from build123d import *

# Parameters (mm, degrees)
SKETCH_1_R          = 7.5
EXTRUDE_1_DEPTH     = 20
SKETCH_2_R          = 3.5
CUT_EXTRUDE_1_DEPTH = 4
SKETCH_3_R          = 1.75
CUT_EXTRUDE_2_DEPTH = 14
SKETCH_4_R          = 1.4
CUT_EXTRUDE_3_DEPTH = 14
SKETCH_5_W          = 18
SKETCH_5_H          = 5
CUT_EXTRUDE_4_DEPTH = 4


with BuildPart() as part:
    # Эскиз1 → Бобышка-Вытянуть1 (new body)
    with BuildSketch(Plane.XY):
        Circle(SKETCH_1_R)
    extrude(amount=EXTRUDE_1_DEPTH)

    # Эскиз2 → Вырез-Вытянуть1 (cut)
    with BuildSketch(Plane.XY.offset(20)):
        Circle(SKETCH_2_R)
    extrude(amount=-CUT_EXTRUDE_1_DEPTH, mode=Mode.SUBTRACT)

    # Эскиз3 → Вырез-Вытянуть2 (cut)
    with BuildSketch(Plane(origin=(0, 0, 0), x_dir=(-1, 0, 0), z_dir=(0, 0, -1))):
        Circle(SKETCH_3_R)
    extrude(amount=-CUT_EXTRUDE_2_DEPTH, mode=Mode.SUBTRACT)

    # Эскиз4 → Вырез-Вытянуть3 (cut)
    with BuildSketch(Plane(origin=(0, 0, 0), x_dir=(1, 0, 0), z_dir=(0, 1, 0))):
        with Locations(Location((0, -7, 0), (0, 0, 270))):
            Circle(SKETCH_4_R)
    extrude(amount=-CUT_EXTRUDE_3_DEPTH, mode=Mode.SUBTRACT)

    # Эскиз5 → Вырез-Вытянуть4 (cut)
    with BuildSketch(Plane.XY.offset(20)):
        Rectangle(SKETCH_5_W, SKETCH_5_H)
    extrude(amount=-CUT_EXTRUDE_4_DEPTH, mode=Mode.SUBTRACT)


solid = part.part
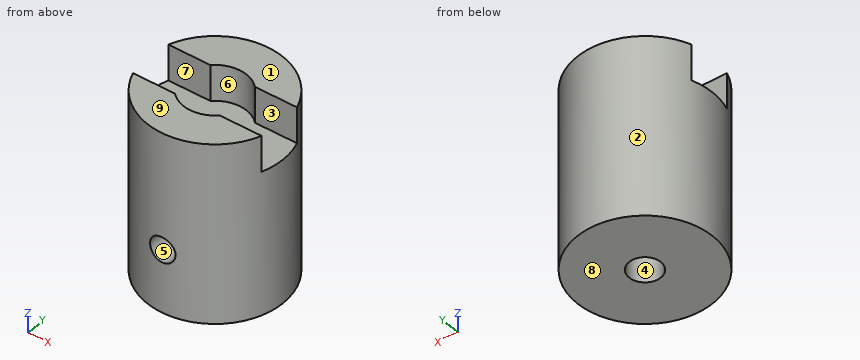
Can you work these out from the model? Positions are in its coordinate system, mm. Face numbers are marked on the shaded views. A direction names the side the tool comes from. Give positions to 0.01 mm unless a question says otherwise; leave off trailing zeros. Write each loop counter-clockwise with the first axis right and the second up, starting at its lowest first coordinate (ties: lowest second). Pieces come first, ordered by that corner, then holes. Notation, with made-up numbers: (53.25, 22) -> (109.25, 22) arc R22 cw to (109.25, 46) -> close; hole circle Ø9 at (55, -6.75). An arc over 180 degrees is marked (long way). Answer as a JSON object with one key per item and string values. Group by question number.
Item 1: For the marked faces 5, 6, 7, 8 and 9, which set-ups out of +Z, -Z, +X, -X, +Y, -Y let a thin tool reach every point of the face, with its end or its side?
Item 2: Suppose I cut it at D-D (x = 6.25). Please give me the cut outline in (y, z), plus the area to 3 significant figures.
Item 3: I'm going to push flat-ended pins straight in: P1, Ø4, axis at x = -2.5, y = 3.5, coming from the -Z side; P2, Ø1, axis at x = 2.5, z = 9.5, coming from the +Y side; P3, Ø2, axis at x = -5, z = 17.5, coming from the -Y side; P4, Ø3, axis at x = -5, z = 17, coming from the +Y side. Where does each tip first touch, or does it pass through?
Item 4: Suppose I cut it at B-B (y = -6). Please give me the cut outline in (x, z).
Item 5: Suppose I cut it at C-C (y = 0). Please give me the cut outline in (x, z), plus the area to 3 significant figures.
Item 6: Please list where these lines run through material, in increasing order: line 1 (Y direction, x = 2.5, z = 18.25); line 2 (Z direction, x = -5, y = -2); line 3 (Z direction, x = 1, y = -4.5). Write a range as [from, to].
Item 7: Suppose I cut it at A-A (x = 0). Please give me the cut outline in (y, z).
Item 8: We'd pull the mould along Y, two halves only. Please class the marked faces 1, 2, 3 and 4: +Y half, -Y half, draft (parallel to the pull), parting line (faces both ways), or undercut.
Findings:
{
 "1": {"face 5": "-Y", "face 6": "+Z", "face 7": "+Z, +X, -X", "face 8": "-Z, +X, -X, +Y, -Y", "face 9": "+Z, +X, -X, +Y, -Y"},
 "2": {"outline": "(-4.15, 0) -> (4.15, 0) -> (4.15, 20) -> (2.5, 20) -> (2.5, 16) -> (-2.5, 16) -> (-2.5, 20) -> (-4.15, 20) -> close", "area": "146 mm²"},
 "3": {"P1": "stops at z = 0", "P2": "stops at y = 7.23", "P3": "stops at y = -6.34", "P4": "stops at y = 6.63"},
 "4": {"outline": "(-4.5, 0) -> (4.5, 0) -> (4.5, 20) -> (-4.5, 20) -> close; hole circle Ø2.8 at (0, 7)"},
 "5": {"outline": "(-7.5, 0) -> (-1.75, 0) -> (-1.75, 14) -> (1.75, 14) -> (1.75, 0) -> (7.5, 0) -> (7.5, 16) -> (-7.5, 16) -> close", "area": "191 mm²"},
 "6": {"line 1": "y = [-7.07, -2.5], [2.5, 7.07]", "line 2": "z = [0, 16]", "line 3": "z = [0, 6.02], [7.98, 20]"},
 "7": {"outline": "(-7.5, 0) -> (-1.75, 0) -> (-1.75, 5.6) -> (-7.5, 5.6) -> close; (-7.5, 8.4) -> (-1.75, 8.4) -> (-1.75, 14) -> (1.75, 14) -> (1.75, 0) -> (7.5, 0) -> (7.5, 20) -> (3.5, 20) -> (3.5, 16) -> (-3.5, 16) -> (-3.5, 20) -> (-7.5, 20) -> close"},
 "8": {"face 1": "draft", "face 2": "parting line", "face 3": "undercut", "face 4": "undercut"}
}
